Here's how the part is built. I have some questions about the finished solid (model axes, mm). Face numbers are marked on the shaded views. Coordinates: 2 decimals unless noted, no trailing zeros. Write each loop counter-clockwise with the first axis right and the second up, starting at its lowest first coordinate (ties: lowest second). Pieces come first, ordered by that corner, then holes.
Item 1: I want a section at C-C (x = 48). Please give me the cut outline in (y, z), and give its area (3 significant figures).
Item 2: If we mould it in two halves opening along X, with no side actions, what happens to the marked faces 1, 2, 3 and 4? For each: pulls with the +X half, pulls with the -X half, needs draft (parallel to the pull), parting line crosses it, or undercut.
Item 3: I want a section at B-B (y = -32). Please give me the cut outline in (x, z), and give its area (4 significant figures).
Item 4: Please list where these lines run through material, in increasing order: line 1 (Y direction, x = -6.5, z = 8); line 2 (X direction, y = 29, z = 4.25); line 3 (Y direction, x = -24, z = 5.5).
Item 5: I'm going to push a flat-ended pin straight in: P1, Ø1.5, axis at x = -37, y = 16, coming from the +Z side. Where does the tip first touch, or does it pass through?
Item 6: I want a section at A-A (z = 6.25). Count the separate pieces of the cut face and the enclosed holes in it, and give its area (3 significant figures).
from build123d import *

# Parameters (mm, degrees)
F0_W     = 127
F0_H     = 86.36
F1_DEPTH = 12.7
F2_T     = -2.54
F3_R     = 1.27
F4_R     = 3.81
F4_R_2   = 2.54
F4_R_3   = 3.987123
F5_DEPTH = 10.16
F4_R_4   = 5.08
F4_R_5   = 5.599952
F6_DEPTH = 5.08
F7_DEPTH = 10.16
F8_DEPTH = 5.08


with BuildPart() as f1:
    # F0 (on Top) → F1 (new body)
    with BuildSketch(Plane.XY):
        Rectangle(F0_W, F0_H)
    extrude(amount=F1_DEPTH)

    # F2
    f2_openings = [f1.faces().sort_by_distance(p)[0] for p in [
        (0, 0, 12.7),
    ]]
    offset(amount=F2_T, openings=f2_openings)

    # F3
    f3_edges = [f1.edges().sort_by_distance(p)[0] for p in [
        (-63.5, 43.18, 6.35),
        (-63.5, 0, 0),
        (0, -43.18, 0),
        (0, 43.18, 0),
        (63.5, 0, 0),
        (63.5, 43.18, 6.35),
        (63.5, -43.18, 6.35),
        (-63.5, -43.18, 6.35),
    ]]
    fillet(f3_edges, radius=F3_R)

    # F4 (on face) → F5 (join)
    with BuildSketch(Plane.XY.offset(2.54)):
        with Locations((-36.485116, 14.837309)):
            Circle(F4_R)
        with Locations((-36.485116, 14.837309)):
            Circle(F4_R_2, mode=Mode.SUBTRACT)
        with Locations((-1.668755, 0.678628)):
            Circle(F4_R_3)
        with Locations((-1.668755, 0.678628)):
            Circle(F4_R_2, mode=Mode.SUBTRACT)
    extrude(amount=F5_DEPTH)

    # F4 (on face) → F6 (join)
    with BuildSketch(Plane.XY.offset(2.54)):
        with Locations((-36.485116, 14.837309)):
            Circle(F4_R_4)
        with Locations((-36.485116, 14.837309)):
            Circle(F4_R, mode=Mode.SUBTRACT)
        with Locations((-1.668755, 0.678628)):
            Circle(F4_R_5)
        with Locations((-1.668755, 0.678628)):
            Circle(F4_R_3, mode=Mode.SUBTRACT)
    extrude(amount=F6_DEPTH)

    # F4 (on face) → F7 (join)
    with BuildSketch(Plane.XY.offset(2.54)):
        with Locations((-19.076936, 7.757969)):
            Circle(F4_R_3)
        with Locations((-19.076936, 7.757969)):
            Circle(F4_R_2, mode=Mode.SUBTRACT)
        with Locations((15.739425, -6.400712)):
            Circle(F4_R_3)
        with Locations((15.739425, -6.400712)):
            Circle(F4_R_2, mode=Mode.SUBTRACT)
    extrude(amount=F7_DEPTH)

    # F4 (on face) → F8 (join)
    with BuildSketch(Plane.XY.offset(2.54)):
        with Locations((-19.076936, 7.757969)):
            Circle(F4_R_5)
        with Locations((-19.076936, 7.757969)):
            Circle(F4_R_3, mode=Mode.SUBTRACT)
        with Locations((15.739425, -6.400712)):
            Circle(F4_R_5)
        with Locations((15.739425, -6.400712)):
            Circle(F4_R_3, mode=Mode.SUBTRACT)
    extrude(amount=F8_DEPTH)


solid = f1.part
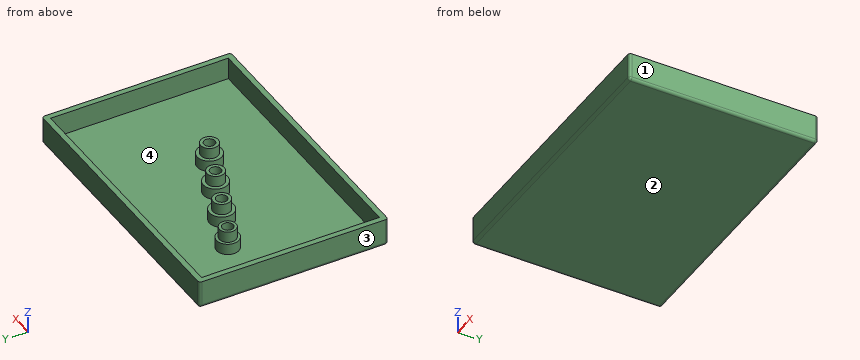
Answer:
1. outline: (-43.18, 1.27) arc R1.27 ccw to (-41.91, 0) - (41.91, 0) arc R1.27 ccw to (43.18, 1.27) - (43.18, 12.7) - (40.64, 12.7) - (40.64, 2.54) - (-40.64, 2.54) - (-40.64, 12.7) - (-43.18, 12.7) - close
1. area: 270 mm2
2. face 1: pulls with the +X half
2. face 2: needs draft
2. face 3: pulls with the -X half
2. face 4: undercut
3. outline: (-63.5, 1.27) arc R1.27 ccw to (-62.23, 0) - (62.23, 0) arc R1.27 ccw to (63.5, 1.27) - (63.5, 12.7) - (60.96, 12.7) - (60.96, 2.54) - (-60.96, 2.54) - (-60.96, 12.7) - (-63.5, 12.7) - close
3. area: 373.5 mm2
4. line 1: y = -43.18 to -40.64, 40.64 to 43.18
4. line 2: x = -63.5 to -60.96, 60.96 to 63.5
4. line 3: y = -43.18 to -40.64, 5.09 to 10.43, 40.64 to 43.18
5. P1: stops at z = 2.54
6. separate pieces: 5
6. enclosed holes: 5
6. area: 1,350 mm2
